Print and shaded views of the part. All mm, measured from the part's lowest x, y and z. Round coordinates to 2 decimals unless told otherwise and drop trailing zeros. Order: outer loops, then holes, each group sorted by start corner. A loop starts at its lowest first (then second) coordinate and runs counter-clockwise, first axis right, second up. Notation, with made-up numbers: M -31,-21.5 L -12,-21.5 A19 ccw -12,-7.5 Z; hole C 21.5,68.5 d11. An arc over 180 degrees is marked long. Use CSV: the item, a comma, the result in double quotes.
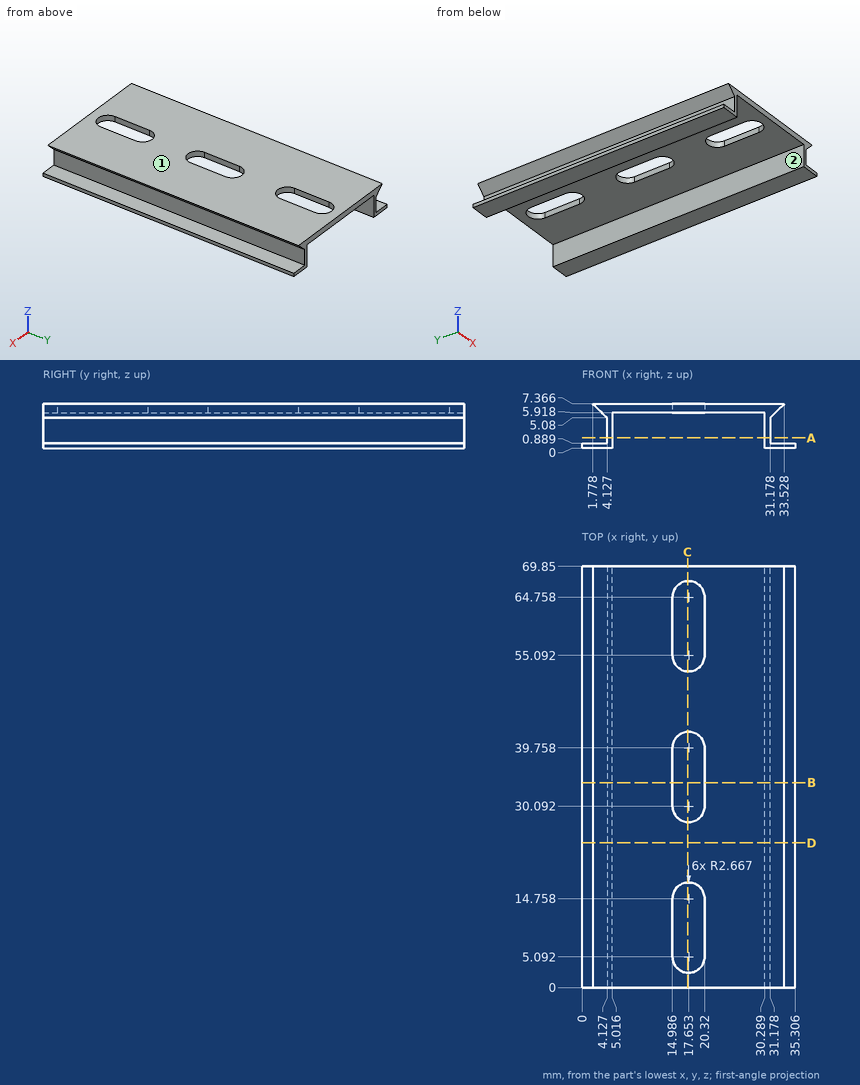
(1) Drop flat-ended pins along their axis: pin 1 (4 mm diameter, centred on x = 16, z = 3, fed in from +Y); pin 2 (3 mm diameter, centred on y = 30.5, z = 2.5, fed in from +X); pin 3 (1.5 mm diameter, centred on y = 42, z = 2, fed in from -X); pin 4 (7.5 mm diameter, centred on x = 17, y = 31, fed in from -Z). Give the stop position or say it passes through.
Answer block:
pin 1,"passes through"
pin 2,"stops at x = 31.18"
pin 3,"stops at x = 4.13"
pin 4,"stops at z = 5.92"
(2) Cut at C-C, the plane x = 17.5. Count the separate pieces of the cut face and the enclosed holes in it.
Answer block:
separate pieces,"4"
enclosed holes,"0"
(3) Wall check: line 1 (X direction, y = 50, z = 0.75) (1 decimal); line 2 (X direction, y = 5.5, z = 1.5); line 3 (Z direction, x = 14.5, y = 11) (1 decimal). Give the ranges that are in metal, low to high. Write a range as from..to.
Answer block:
line 1,"x = 0..5, 30.3..35.3"
line 2,"x = 4.13..5.02, 30.29..31.18"
line 3,"z = 5.9..7.4"
(4) Cut at A-A, the plane z = 1.75. Give the cut face in (x, y), and give its area (3 significant figures).
Answer block:
outline,"M 4.13,0 L 5.02,0 L 5.02,69.85 L 4.13,69.85 Z; M 30.29,0 L 31.18,0 L 31.18,69.85 L 30.29,69.85 Z"
area,"124 mm²"
(5) Cut at B-B, the plane y = 34. Give the cut face in (x, z) (1 decimal).
Answer block:
outline,"M 0,0 L 5,0 L 5,5.9 L 15,5.9 L 15,7.4 L 1.8,7.4 L 4.1,5.1 L 4.1,0.9 L 0,0.9 Z; M 20.3,5.9 L 30.3,5.9 L 30.3,0 L 35.3,0 L 35.3,0.9 L 31.2,0.9 L 31.2,5.1 L 33.5,7.4 L 20.3,7.4 Z"
(6) Two-plate mould, pull along X, no slides. Class the marked faces 1 and 2: released by +X, released by -X, zero draft, split by the parting line, or undercut.
Answer block:
face 1,"zero draft"
face 2,"undercut"
(7) Cut at D-D, the plane y = 24. Give the cut face in (x, z) (1 decimal).
Answer block:
outline,"M 0,0 L 5,0 L 5,5.9 L 30.3,5.9 L 30.3,0 L 35.3,0 L 35.3,0.9 L 31.2,0.9 L 31.2,5.1 L 33.5,7.4 L 1.8,7.4 L 4.1,5.1 L 4.1,0.9 L 0,0.9 Z"
